Work out the finished part from the listing and answer in its coordinate system (mm). A direction names the side the tool comes from. Coordinates: 2 decimals unless noted, no trailing zeros. Order: outer loops, then holes, each group sorted by start corner. A loop starts at its lowest first (then second) coordinate and runs counter-clockwise, first axis right, second up. Notation, with made-up numbers: M -3.75,-26.5 L 20.25,-26.5 A36 ccw 20.25,7.5 Z; hole C -6.75,50 d4. An arc over 180 degrees is marked long. Answer in a Markdown table with one row per item. Add a question column.
Item 1: The part is cut by section B-B (z = -11.5). Write down the section's boundary in (x, y).
Item 2: The part is cut by section A-A (x = 2.5). Write down the section's boundary in (y, z), then the cut area to 3 significant figures.
Item 3: The part is cut by section C-C (y = 1.25). Write down the section's boundary in (x, z).
Item 4: Consider line 1 (Z direction, x = 2.5, y = 0.9); line 2 (X direction, y = 1.35, z = -11.5); line 3 (Z direction, x = 5.75, y = 1.25). Determine where each line is inside the solid, lowest interval first. Write a range as from..to.
Item 5: Flat-ended cylindrical pins translate along their axes: pin 1 Ø1 at (y, z) = (0.5, -4) entering from +X; pin 2 Ø0.8 at (x, y) = (-0.5, 1) entering from +Z; pin 3 Ø0.6 at (y, z) = (1.5, -4.5) entering from -X. Find the tip coordinate at first contact, or state that the pin passes through.
Item 6: The mould has two halves that part along X. Classify faces 4 (the face through (-0.5, 1, -7)), 5 (the face through (3.172, 1.014, -12.554)), 6 (the face through (5, 1, -3)): released by +X, released by -X, zero draft, split by the parting line, or undercut.
Item 7: The part is cut by section D-D (z = -2). Write down the section's boundary in (x, y), then the cut area to 3 significant figures.
Item 8: Which of the six approach directions +Z, -Z, +X, -X, +Y, -Y give full straight-line access (tool end or side, diameter ignored) to faces 1 (the face through (5.5, 1, -7)), 2 (the face through (0, 1, -3)), 3 (the face through (2, 1, 0))?
Autodesk Inventor part; units mm, degrees
ref_plane "YZ Plane" through (0, 0, 0) normal (1, 0, 0) x (0, 1, 0)
ref_plane "XZ Plane" through (0, 0, 0) normal (0, 1, 0) x (-1, 0, 0)
ref_plane "XY Plane" through (0, 0, 0) normal (0, 0, 1) x (1, 0, 0)
sketch "Sketch3" plane through (0, 0, 0) normal (0, 1, 0) x (-1, 0, 0)
  line L0 (0, 0) -> (-5, 0)
  line L1 (-5, 0) -> (-5, -7)
  line L2 (0, 0) -> (0, -7)
  line L3 (0, -7) -> (1, -7)
  line L4 (1, -7) -> (1, -15)
  line L5 (-5, -7) -> (-6, -7)
  line L6 (-6, -7) -> (-6, -15)
  line L7 (-6, -15) -> (1, -15)
  dimension "d9" = 5
  dimension "d10" = 7
  dimension "d11" = 1
  dimension "d12" = 8
  dimension "d13" = 1
extrude "Extrusion3" add sketch "Sketch3" along normal blind 2
sketch "Sketch4" plane through (0, 2, 0) normal (0, 1, 0) x (1, 0, 0)
  line L0 (-1, 15) -> (-1, 7)
  line L1 (-1, 15) -> (2.5, 15)
  line L2 (6, 15) -> (-1, 15)
  line L3 (2.5, 15) -> (2.5, 11.5)
  circle A0 centre (2.5, 11.5) radius 1.25
  point P0 (0, 0)
  dimension "d16" = 3.5
  dimension "d17" = 3.5
  dimension "d18" = 2.5
extrude "Extrusion4" cut sketch "Sketch4" against normal blind 2
properties part number "HINGE A"
Reply:
| question | item | result |
|---|---|---|
| 1 | outline | M -1,0 L 1.25,0 L 1.25,2 L -1,2 Z; M 3.75,0 L 6,0 L 6,2 L 3.75,2 Z |
| 2 | outline | M 0,-15 L 2,-15 L 2,-12.75 L 0,-12.75 Z; M 0,-10.25 L 2,-10.25 L 2,0 L 0,0 Z |
| 2 | area | 25.0 mm2 |
| 3 | outline | M -1,-15 L 6,-15 L 6,-7 L 5,-7 L 5,0 L 0,0 L 0,-7 L -1,-7 Z; hole C 2.5,-11.5 d2.5 |
| 4 | line 1 | z = -15..-12.75, -10.25..0 |
| 4 | line 2 | x = -1..1.25, 3.75..6 |
| 4 | line 3 | z = -15..-7 |
| 5 | pin 1 | stops at x = 5 |
| 5 | pin 2 | stops at z = -7 |
| 5 | pin 3 | stops at x = 0 |
| 6 | face 4 | zero draft |
| 6 | face 5 | undercut |
| 6 | face 6 | released by +X |
| 7 | outline | M 0,0 L 5,0 L 5,2 L 0,2 Z |
| 7 | area | 10.0 mm2 |
| 8 | face 1 | +Z, +X, +Y, -Y |
| 8 | face 2 | +Z, -X, +Y, -Y |
| 8 | face 3 | +Z, +X, -X, +Y, -Y |
